from build123d import *

# Parameters (mm, degrees)
F0_W     = 203.2
F0_H     = 101.6
F1_DEPTH = 50.8
F2_W     = 50.8
F2_H     = 50.8
F3_DEPTH = 101.6
F4_ANGLE = 180


with BuildPart() as f1:
    # F0 (on Top) → F1 (new body)
    with BuildSketch(Plane.XY):
        with Locations((8.5724983364, -10.0287537194)):
            Rectangle(F0_W, F0_H)
    extrude(amount=F1_DEPTH)

    # F2 (on face) → F3 (join)
    with BuildSketch(Plane(origin=(0, 40.7712462806, 0), x_dir=(-1, 0, 0), z_dir=(0, 1, 0))):
        with Locations((-84.7724983364, 76.2)):
            Rectangle(F2_W, F2_H)
    extrude(amount=-F3_DEPTH)


with BuildPart() as f1_1:
    # F4: moved
    add(f1.part.rotate(Axis((110.1724983364, -60.8287537194, 25.4), (0, 0, -1)), F4_ANGLE))


solid = f1_1.part
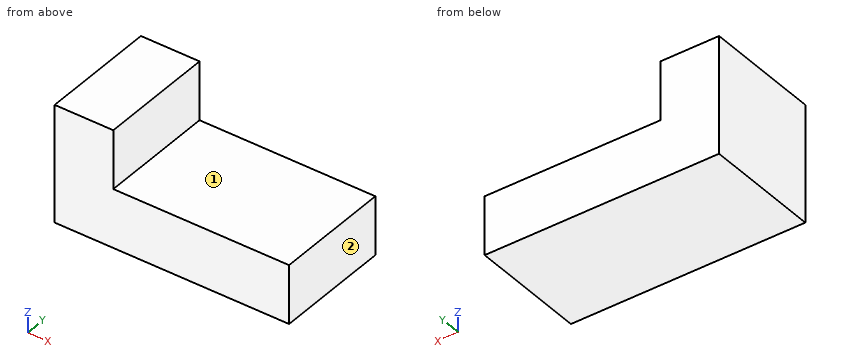
Verification items for the finished model (mm, model axes). Face numbers are marked on the shaded views. A direction names the side the tool comes from. Round coordinates to 2 decimals unless told otherwise and drop trailing zeros. Loops run counter-clockwise (first coordinate to the right, second up) from the corner with the lowest first, then second, coordinate; pieces in that order, holes last. Notation, with made-up numbers: (26.5, -17) - (73.5, -17) arc R28 ccw to (73.5, 14) - close; hole circle Ø11 at (-24.5, 27). An arc over 180 degrees is marked (long way). Use one line per item in the form item = value.
1. Section check A-A on x = 262.5. Record the cut outline in (y, z).
A:
outline = (-162.43, 0) - (-60.83, 0) - (-60.83, 50.8) - (-162.43, 50.8) - close
2. Scan lines: probe 1 along Z at (x, y) = (273.5, -105); probe 2 along X at (y, z) = (-82.5, 95). Record each from-to range of solid material in increasing order.
A:
probe_1 = 0 to 50.8
probe_2 = 110.17 to 160.97
3. Section check C-C on y = -147.5. Record the cut outline in (x, z), and give its area (3 significant figures).
A:
outline = (110.17, 0) - (313.37, 0) - (313.37, 50.8) - (160.97, 50.8) - (160.97, 101.6) - (110.17, 101.6) - close
area = 12,900 mm²
4. Access from +Z, -Z, +X, -X, +Y, -Y to the whole of each face (thin tool, end or side, straight path). Record for the marked faces 1 and 2.
A:
face_1 = +Z, +X, +Y, -Y
face_2 = +Z, -Z, +X, +Y, -Y
5. Section check B-B on z = 83. Record the cut outline in (x, y), and give its area (3 significant figures).
A:
outline = (110.17, -162.43) - (160.97, -162.43) - (160.97, -60.83) - (110.17, -60.83) - close
area = 5,160 mm²
6. Gauge pin test, flat end, axial feed: pin 1 Ø1 at (x, y) = (243.5, -86.5) entering from +Z. Record the tip position at first contact, or that the pin passes through.
A:
pin_1 = 50.8
